Can you work these out from the model? Positions are in its coordinate system, mm. Face numbers are marked on the shaded views. Give positions to 0.01 mm unless a question says otherwise; leave off trailing zeros. Write each loop counter-clockwise with the first axis right and the second up, starting at its lowest first coordinate (ties: lowest second). Pieces come first, ordered by that corner, then holes. Notation, with made-up numbers: (62, 85.5) -> (70, 85.5) arc R4 cw to (70, 89.5) -> close; hole circle Ø5 at (37, 25). An arc over 180 degrees is marked (long way). One line per item, written item: value.
from build123d import *

# Parameters (mm, degrees)
SKETCH1_W                                 = 15
SKETCH1_H                                 = 25
BOSS_EXTRUDE1_DEPTH                       = 4
SKETCH2_W                                 = 15
SKETCH2_H                                 = 4
BOSS_EXTRUDE2_DEPTH                       = 22
M5X0_8_TAPPED_HOLE2_D                     = 4.2
M5X0_8_TAPPED_HOLE2_CSINK_D               = 5.05
M5X0_8_TAPPED_HOLE2_CSINK_ANGLE           = 90
M5X0_8_TAPPED_HOLE2_ON_FACE_2_D           = 4.2
M5X0_8_TAPPED_HOLE2_ON_FACE_2_CSINK_D     = 5.05
M5X0_8_TAPPED_HOLE2_ON_FACE_2_CSINK_ANGLE = 90


with BuildPart() as part:
    # Sketch1 → Boss-Extrude1 (new body)
    with BuildSketch(Plane(origin=(0, 0, 0), x_dir=(1, 0, 0), z_dir=(0, 1, 0))):
        with Locations((-22.468152866, 0.119426752)):
            Rectangle(SKETCH1_W, SKETCH1_H)
    extrude(amount=BOSS_EXTRUDE1_DEPTH)

    # Sketch2 → Boss-Extrude2 (add)
    with BuildSketch(Plane(origin=(0, 4, 0), x_dir=(1, 0, 0), z_dir=(0, 1, 0))):
        with Locations((-22.468152866, 10.619426752)):
            Rectangle(SKETCH2_W, SKETCH2_H)
    extrude(amount=BOSS_EXTRUDE2_DEPTH)

    # M5x0.8 Tapped Hole2 (through all)
    with Locations(Plane(origin=(-22.703417576, 4, 2.485289676), x_dir=(0, 0, 1), z_dir=(0, 1, 0))):
        with Locations((0, 0)):
            CounterSinkHole(M5X0_8_TAPPED_HOLE2_D / 2, M5X0_8_TAPPED_HOLE2_CSINK_D / 2, counter_sink_angle=M5X0_8_TAPPED_HOLE2_CSINK_ANGLE)

    # M5x0.8 Tapped Hole2 on face 2 (through all)
    with Locations(Plane(origin=(-22.76831123, 14.89235582, -8.619426752), x_dir=(1, 0, 0), z_dir=(0, 0, 1))):
        with Locations((0, 0)):
            CounterSinkHole(M5X0_8_TAPPED_HOLE2_ON_FACE_2_D / 2, M5X0_8_TAPPED_HOLE2_ON_FACE_2_CSINK_D / 2, counter_sink_angle=M5X0_8_TAPPED_HOLE2_ON_FACE_2_CSINK_ANGLE)


solid = part.part
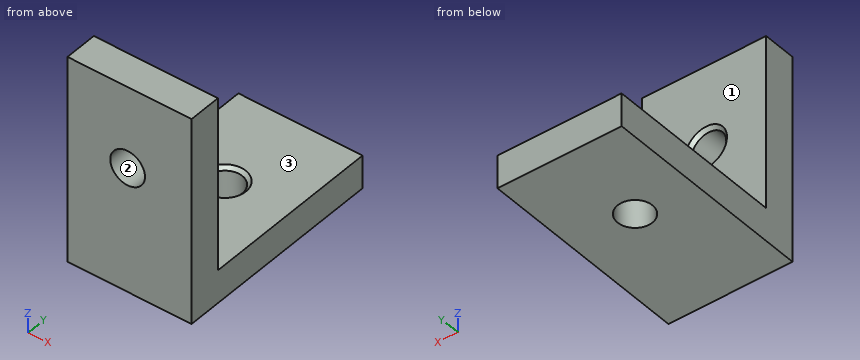
1) If we section it at A-A (x = -18): Write out the boundary of the cut face in (y, z), and give its area (3 significant figures).
Answer list:
outline: (0, -12.62) -> (26, -12.62) -> (26, -8.62) -> (4, -8.62) -> (4, 12.38) -> (0, 12.38) -> close
area: 188 mm^2
2) If we section it at D-D (x = -23.25): State how many separate pieces and enclosed holes the cut face has, and give its area (3 significant figures).
Answer list:
separate pieces: 3
enclosed holes: 0
area: 155 mm^2
3) We'd pull the mould along Z, two halves only. Please class the marked faces 1, 2 and 3: released by +Z, released by -Z, zero draft, split by the parting line, or undercut.
Answer list:
face 1: zero draft
face 2: undercut
face 3: released by +Z
4) Will these pins go through, and if not, where does the flat tip stop? pin 1 (10 mm diameter, centred on y = 10.5, z = -8.5, fed in from -X); pin 2 (1.5 mm diameter, centred on x = -18, z = -4, fed in from +Y); pin 3 (7.5 mm diameter, centred on x = -19, y = 14, fed in from +Z).
Answer list:
pin 1: stops at x = -29.97
pin 2: stops at y = 4
pin 3: stops at z = -8.62
5) I need wall thicknesses on L1, parallel to Y at x = -18, z = -4.75; L2, parallel to Z at x = -24.75, y = 9.5; L3, parallel to X at y = 15.5, z = -10. Which ranges of each line are inside material? Lowest first, please.
Answer list:
L1: y = 0 to 4
L2: z = -12.62 to -8.62
L3: x = -29.97 to -24.78, -20.76 to -14.97
6) If we section it at B-B (y = 19.25): Write out the boundary of the cut face in (x, z), and give its area (3 significant figures).
Answer list:
outline: (-29.97, -12.62) -> (-14.97, -12.62) -> (-14.97, -8.62) -> (-29.97, -8.62) -> close
area: 60.0 mm^2
7) If we section it at C-C (z = -10): Write out the boundary of the cut face in (x, y), and give its area (3 significant figures).
Answer list:
outline: (-29.97, 0) -> (-14.97, 0) -> (-14.97, 26) -> (-29.97, 26) -> close; hole circle Ø4.2 at (-22.77, 14.89)
area: 376 mm^2
